Could you check a few things on this model? Use its own coordinates, in mm. A direction names the side the tool comes from. Round coordinates to 2 decimals unless told otherwise and drop trailing zeros. Loops run counter-clockwise (first coordinate to the right, second up) from the corner with the lowest first, then second, coordinate; pieces in that order, holes last. Notation, with made-up numbers: M -15.5,50 L 34.5,50 A22 cw 34.5,73 Z; hole C 35.5,62.25 d11. An arc over 180 degrees is marked long. One line per item, written item: value. Start each with the question number.
Q1. Imagine slicing it at A-A (z = 0). Please give me the cut outline in (x, y), then the cut area to 3 significant figures.
Q2. Imagine slicing it at D-D (x = 2). Please give me the cut outline in (y, z), then the cut area to 3 significant figures.
Q3. Which directions (+Z, -Z, +X, -X, +Y, -Y) give clear straight access to the entire face, cutting with the end or side of a thin tool? Please do faces 4 (the face through (4.4, 3.1, -0.994)), 5 (the face through (4, 0, 2)).
Q4. Please list where these lines run through material, in increasing order: line 1 along Z through (x, y) = (0, 4.2); line 2 along Z through (x, y) = (0, 1); line 3 along Y through (x, z) = (-0.5, -1).
Q5. Thinking about a two-plate mould opening in X: for faces 1 (the face through (0, 5.5, 0)), 2 (the face through (-3.797, 4.507, -0.153)), 3 (the face through (5.774, 3, 0)), which applies, released by +X, released by -X, zero draft, split by the parting line, or undercut?
Q6. I'm going to push flat-ended pins straight in: pin 1 Ø0.5 at (x, y) = (4, 3) entering from -Z; pin 2 Ø1 at (x, y) = (3, 4) entering from -Z; pin 3 Ø2 at (x, y) = (2.5, 1.5) entering from -Z. Where does each tip first touch, or does it pass through?
Q7. Imagine slicing it at C-C (x = 0). Please give me the cut outline in (y, z).
Q8. Imagine slicing it at B-B (y = 3.35). Please give me the cut outline in (x, z), then the cut area to 3 significant figures.
from build123d import *

# Parameters (mm, degrees)
BOSS_EXTRUDE1_DEPTH = 5
BOSS_EXTRUDE2_DEPTH = 0.5
BOSS_EXTRUDE3_DEPTH = 1


with BuildPart() as part:
    # Sketch1 → Boss-Extrude1 (new body)
    with BuildSketch(Plane(origin=(0, 0, 0), x_dir=(1, 0, 0), z_dir=(0, 1, 0))):
        with BuildLine():
            ThreePointArc((4.566687335, 1.478298611), (-4.8, 0), (4.566687335, -1.478298611))
            ThreePointArc((4.566687335, -1.478298611), (5.403490366, -1.276916974), (5.773887305, -0.5))
            Line((5.773887305, -0.5), (5.773887305, 0.5))
            ThreePointArc((5.773887305, 0.5), (5.403490366, 1.276916974), (4.566687335, 1.478298611))
        make_face()
        with BuildLine():
            ThreePointArc((5.273887305, -0.5), (5.098728559, -0.880102828), (4.695974666, -0.993892317))
            Line((4.695974666, -0.993892317), (4.183560453, -0.993892317))
            ThreePointArc((4.183560453, -0.993892317), (-4.3, 0), (4.183560453, 0.993892317))
            Line((4.183560453, 0.993892317), (4.695974666, 0.993892317))
            ThreePointArc((4.695974666, 0.993892317), (5.098728559, 0.880102828), (5.273887305, 0.5))
            Line((5.273887305, 0.5), (5.273887305, -0.5))
        make_face(mode=Mode.SUBTRACT)
    extrude(amount=BOSS_EXTRUDE1_DEPTH)

    # Sketch3 → Boss-Extrude2 (add)
    with BuildSketch(Plane(origin=(0, 5, 0), x_dir=(1, 0, 0), z_dir=(0, 1, 0))):
        with BuildLine():
            Line((5.773887305, -0.5), (5.773887305, 0.5))
            ThreePointArc((5.773887305, 0.5), (5.403490366, 1.276916974), (4.566687335, 1.478298611))
            ThreePointArc((4.566687335, 1.478298611), (-4.8, 0), (4.566687335, -1.478298611))
            ThreePointArc((4.566687335, -1.478298611), (5.403490366, -1.276916974), (5.773887305, -0.5))
        make_face()
    extrude(amount=BOSS_EXTRUDE2_DEPTH)

    # Sketch4 → Boss-Extrude3 (add)
    with BuildSketch(Plane.XZ.offset(-5)):
        with BuildLine():
            Line((3.667721099, 0.993892317), (4.183560453, 0.993892317))
            ThreePointArc((4.183560453, 0.993892317), (-4.3, 0), (4.183560453, -0.993892317))
            Line((4.183560453, -0.993892317), (3.667721099, -0.993892317))
            ThreePointArc((3.667721099, -0.993892317), (-3.8, 0), (3.667721099, 0.993892317))
        make_face()
    extrude(amount=BOSS_EXTRUDE3_DEPTH)


solid = part.part
Report:
1. outline: M -4.8,0 L -4.3,0 L -4.3,4 L -3.8,4 L -3.8,5 L 5.27,5 L 5.27,0 L 5.77,0 L 5.77,5.5 L -4.8,5.5 Z
1. area: 10.8 mm²
2. outline: M 0,-4.36 L 5.5,-4.36 L 5.5,4.36 L 0,4.36 L 0,3.81 L 4,3.81 L 4,3.23 L 5,3.23 L 5,-3.23 L 4,-3.23 L 4,-3.81 L 0,-3.81 Z
2. area: 11.1 mm²
3. face 4: -Y
3. face 5: +Z, -Z, +X, -X, -Y
4. line 1: z = -4.8 to -3.8, 3.8 to 4.8
4. line 2: z = -4.8 to -4.3, 4.3 to 4.8
4. line 3: y = 5 to 5.5
5. face 1: zero draft
5. face 2: undercut
5. face 3: released by +X
6. pin 1: stops at z = -3
6. pin 2: stops at z = -4.1
6. pin 3: stops at z = -4.56
7. outline: M 0,-4.8 L 5.5,-4.8 L 5.5,4.8 L 0,4.8 L 0,4.3 L 4,4.3 L 4,3.8 L 5,3.8 L 5,-3.8 L 4,-3.8 L 4,-4.3 L 0,-4.3 Z
8. outline: M 4.57,-1.48 A1 ccw 5.77,-0.5 L 5.77,0.5 A1 ccw 4.57,1.48 A4.8 ccw long Z; hole M 4.18,-0.99 L 4.7,-0.99 A0.5 ccw 5.27,-0.5 L 5.27,0.5 A0.5 ccw 4.7,0.99 L 4.18,0.99 A4.3 ccw long Z
8. area: 15.1 mm²
